Check sheet for the drawn part. Datum: minimum x, y, z corner. Units: mm. A direction names the side the tool comes from. Round coordinates to 2 decimals unless told otherwise and drop trailing zeros. Order: outer loops, then holes, each group sorted by start corner. A loop starts at its lowest first (then second) coordinate and runs counter-clockwise, first axis right, second up. Notation, with made-up numbers: M 10,56 L 37,56 A32 ccw 37,90 Z; hole C -23,7 d9. An arc over 180 degrees is marked long. Use one line per item in the form item = value. Start each with the question number.
Item 1: Go/stop test with flat-tipped pins: pin 1 Ø1.1 at (x, y) = (14.5, 2.5) entering from -Z; pin 2 Ø1.5 at (x, y) = (13, 0.5) entering from +Z; pin 3 Ø6.5 at (x, z) = (9.5, 7.5) entering from -Y; pin 4 Ø0.8 at (x, y) = (14.5, 2.5) entering from +Z. Record where each tip stops, or that it passes through.
Item 2: Cross-section at D-D on y = 0.3. Enter the section's corners in (x, z), then the cut area to 3 significant figures.
Item 3: Tool access check on the marked faces 1 and 2. Record the directions out of +Z, -Z, +X, -X, +Y, -Y that give a thin tool (end or side, any length) a straight path to the whole face; none if there is none.
Item 4: Thickness scan on probe 1 along X at (y, z) = (2.7, 6.25); probe 2 along Y at (x, z) = (3, 9.25); probe 3 along Y at (x, z) = (6.25, 6.75). Record the ranges inside material, lowest first. Write a range as [from, to].
Item 5: Cross-section at A-A on y = 2.1. Enter the section's corners in (x, z).
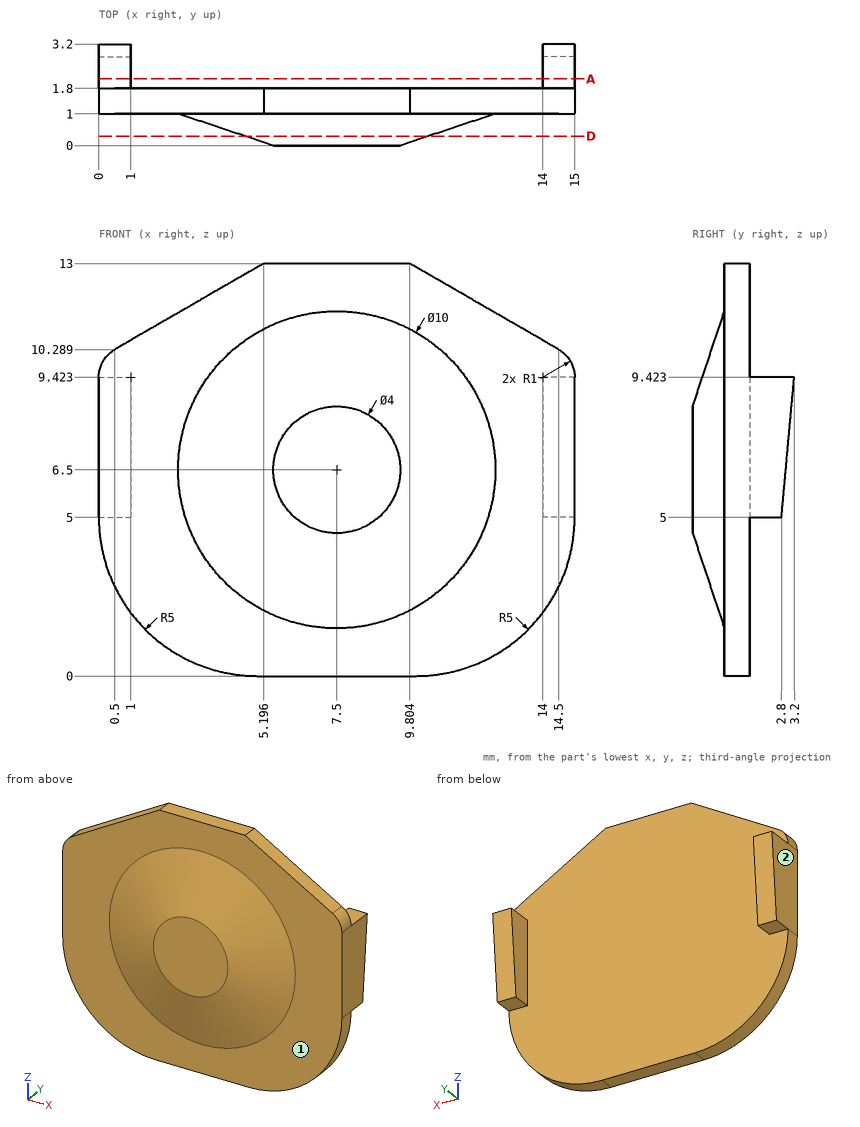
Output values:
q1.pin_1 = 5
q1.pin_2 = 11.48
q1.pin_3 = 0
q1.pin_4 = 9.42
q2.outline = C 7.5,6.5 d5.8
q2.area = 26.4 mm2
q3.face_1 = -Y
q3.face_2 = +Z, -Z, -X, +Y, -Y
q4.probe_1 = [0, 1], [14, 15]
q4.probe_2 = [1, 1.8]
q4.probe_3 = [0, 1.8]
q5.outline = M 0,5 L 1,5 L 1,9.42 L 0,9.42 Z; M 14,5 L 15,5 L 15,9.42 L 14,9.42 Z
